from build123d import *

# Parameters (mm, degrees)
SKETCH1_W           = 70
SKETCH1_H           = 15
BOSS_EXTRUDE1_DEPTH = 1.5
SKETCH2_W           = 1.5
SKETCH2_H           = 15
BOSS_EXTRUDE2_DEPTH = 22
SKETCH3_R           = 1.5
CUT_EXTRUDE1_DEPTH  = 71


with BuildPart() as part:
    # Sketch1 → Boss-Extrude1 (new body)
    with BuildSketch(Plane(origin=(0, 0, 0), x_dir=(1, 0, 0), z_dir=(0, 1, 0))):
        Rectangle(SKETCH1_W, SKETCH1_H)
    extrude(amount=BOSS_EXTRUDE1_DEPTH)

    # Sketch2 → Boss-Extrude2 (add)
    with BuildSketch(Plane(origin=(0, 1.5, 0), x_dir=(1, 0, 0), z_dir=(0, 1, 0))):
        with Locations((-34.25, 0)):
            Rectangle(SKETCH2_W, SKETCH2_H)
        with Locations((34.25, 0)):
            Rectangle(SKETCH2_W, SKETCH2_H)
    extrude(amount=BOSS_EXTRUDE2_DEPTH)

    # Sketch3 → Cut-Extrude1 (cut, through all)
    with BuildSketch(Plane.ZY.offset(35)):
        with BuildLine():
            Line((7.5, 23.5), (0, 23.5))
            ThreePointArc((0, 23.5), (5.303300859, 21.303300859), (7.5, 16))
            Line((7.5, 16), (7.5, 23.5))
        make_face()
        with BuildLine():
            Line((-7.5, 23.5), (-7.5, 16))
            ThreePointArc((-7.5, 16), (-5.303300859, 21.303300859), (0, 23.5))
            Line((0, 23.5), (-7.5, 23.5))
        make_face()
        with Locations((0, 16)):
            Circle(SKETCH3_R)
    extrude(amount=-CUT_EXTRUDE1_DEPTH, mode=Mode.SUBTRACT)


solid = part.part
Could you check a few things on this model? Use its own coordinates, in mm. A direction names the side the tool comes from. Give positions to 0.01 mm unless a question says otherwise; leave off trailing zeros. Order: outer loops, then holes, each group sorted by start corner. A loop starts at its lowest first (then second) coordinate and runs counter-clockwise, first axis right, second up. Notation, with made-up numbers: (28.5, 65.25) - (50.5, 65.25) arc R34 ccw to (50.5, 104.25) - close; hole circle Ø10 at (23, 12.25). An arc over 180 degrees is marked (long way). Return JSON: item names as keys, results as strings. Group by question number.
Q1. Which directions (+Z, -Z, +X, -X, +Y, -Y) give clear straight access to the entire face, cutting with the end or side of a thin tool? Please do faces 1 (the face through (-35, 12, 0)), 2 (the face through (-33.5, 12, 0)).
Q2. Suppose I cut it at A-A, the plane y = 7.5. Please give me the cut outline in (x, z).
Q3. Please list where these lines run through material, in increasing order: line 1 along Y through (x, z) = (34.45, 0); line 2 along X through (y, z) = (5.5, -0.25); line 3 along Y through (x, z) = (0, 5). Write a range as [from, to].
Q4. Suppose I cut it at C-C, the plane x = -11. Please give me the cut outline in (y, z), and give its area (3 significant figures).
Q5. Thinking about a two-plate mould opening in Z: for faces 3 (the face through (0, 1, 7.5)), 4 (the face through (0, 1.5, 0)), 5 (the face through (-34.26, 17.01, -1.11)), 6 (the face through (34.24, 17.01, -1.11)), which applies, pulls with the +Z half, pulls with the -Z half, needs draft (parallel to the pull), parting line crosses it, or undercut?
Q6. Suppose I cut it at B-B, the plane z = 5.75. Please give me the cut outline in (x, y).
Q7. Will these pins go through, and if not, where does the flat tip stop? pin 1 Ø2.5 at (y, z) = (16, 0) entering from +X; pin 2 Ø8 at (x, z) = (23, -4.5) entering from +Y.
Q8. Suppose I cut it at D-D, the plane y = 18.5. Please give me the cut outline in (x, z), and give its area (3 significant figures).
Resolved:
{
 "1": {"face 1": "+Z, -Z, -X, +Y, -Y", "face 2": "+Z, -Z, +Y"},
 "2": {"outline": "(-35, -7.5) - (-33.5, -7.5) - (-33.5, 7.5) - (-35, 7.5) - close; (33.5, -7.5) - (35, -7.5) - (35, 7.5) - (33.5, 7.5) - close"},
 "3": {"line 1": "y = [0, 14.5], [17.5, 23.5]", "line 2": "x = [-35, -33.5], [33.5, 35]", "line 3": "y = [0, 1.5]"},
 "4": {"outline": "(0, -7.5) - (1.5, -7.5) - (1.5, 7.5) - (0, 7.5) - close", "area": "22.5 mm2"},
 "5": {"face 3": "pulls with the +Z half", "face 4": "needs draft", "face 5": "undercut", "face 6": "undercut"},
 "6": {"outline": "(-35, 0) - (35, 0) - (35, 20.82) - (33.5, 20.82) - (33.5, 1.5) - (-33.5, 1.5) - (-33.5, 20.82) - (-35, 20.82) - close"},
 "7": {"pin 1": "passes through", "pin 2": "stops at y = 1.5"},
 "8": {"outline": "(-35, -7.07) - (-33.5, -7.07) - (-33.5, 7.07) - (-35, 7.07) - close; (33.5, -7.07) - (35, -7.07) - (35, 7.07) - (33.5, 7.07) - close", "area": "42.4 mm2"}
}
